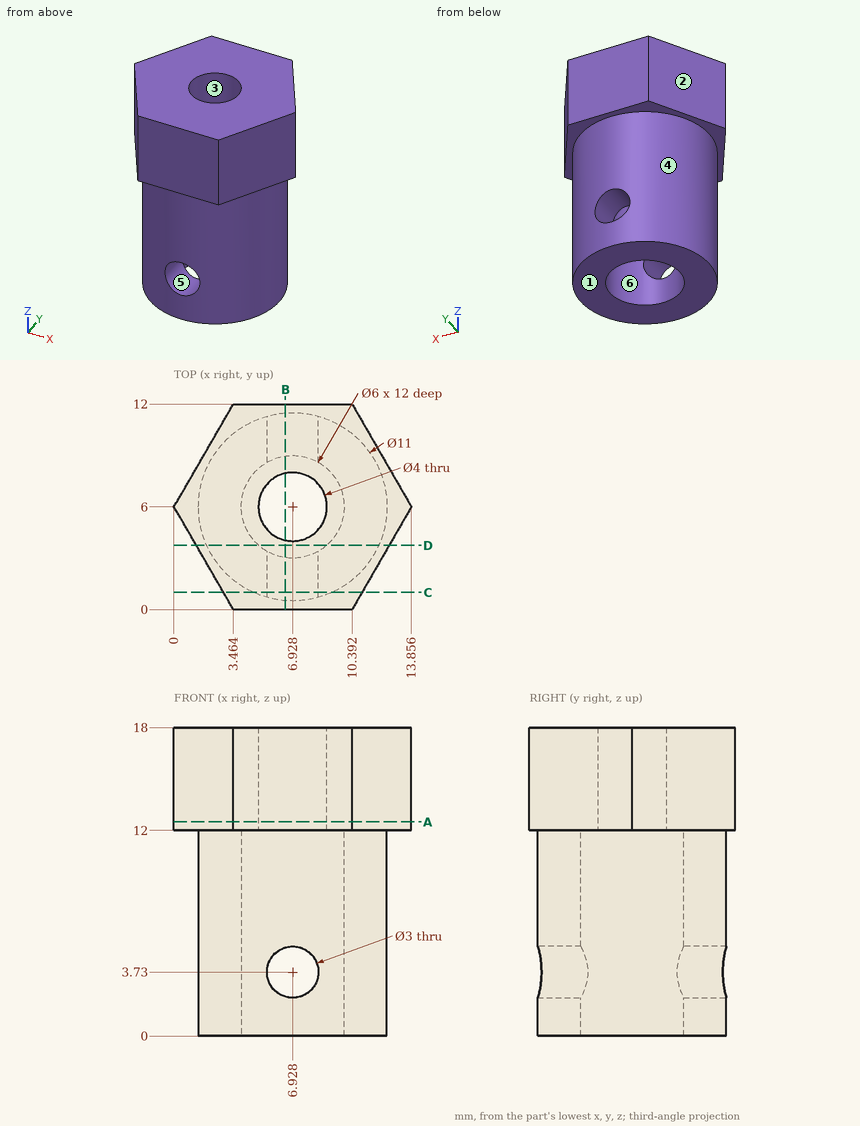
Check sheet for the drawn part. Datum: minimum x, y, z corner. Units: mm. A direction names the side the tool comes from. Give positions to 0.01 mm unless a question says otherwise; leave off trailing zeros. Write each loop counter-clockwise with the first axis right and the second up, starting at its lowest first coordinate (ties: lowest second). Pieces come first, ordered by that corner, then holes.
(1) Material ranges on line 1 (X direction, y = 5, z = 1); line 2 (Z direction, x = 8.25, y = 11); line 3 (Z direction, x = 5.75, y = 11), recorded low to high.
(2) Cross-section at D-D (y = 3.75). Enter the section's corners in (x, z).
(3) Gauge pin test, flat ends, axial feed: pin 1 (5 mm diameter, centred on x = 6.93, y = 6, fed in from -Z); pin 2 (5 mm diameter, centred on x = 6.93, z = 3.73, fed in from -Y); pin 3 (3 mm diameter, centred on y = 7, z = 16, fed in from -X); pin 4 (3.5 mm diameter, centred on x = 6.93, y = 6, fed in from +Z). Record the tip position at first contact, or that the pin passes through.
(4) Mould release check, pull along X, two halves, no side actions. Record for the marked faces 1, 2, 3 and 4: +X half, -X half, draft (parallel to the pull), parting line (faces both ways), or undercut.
(5) Cross-section at C-C (y = 1). Enter the section's corners in (x, z).
(6) Cross-section at A-A (z = 12.5). Enter the section's corners in (x, y), plus the area to 3 significant figures.
(7) Cross-section at B-B (x = 6.5). Enter the section's corners in (y, z).
(8) Access from +Z, -Z, +X, -X, +Y, -Y to the whole of each face (thin tool, end or side, straight path). Record for the marked faces 5 and 6.
Worked out:
1. line 1: x = 1.52 to 4.1, 9.76 to 12.34
1. line 2: z = 0 to 3.02, 4.44 to 18
1. line 3: z = 0 to 2.8, 4.66 to 18
2. outline: (1.3, 12) - (1.91, 12) - (1.91, 0) - (4.94, 0) - (4.94, 12) - (8.91, 12) - (8.91, 0) - (11.95, 0) - (11.95, 12) - (12.56, 12) - (12.56, 18) - (1.3, 18) - close
3. pin 1: stops at z = 12
3. pin 2: stops at y = 0.5
3. pin 3: stops at x = 0
3. pin 4: passes through
4. face 1: draft
4. face 2: -X half
4. face 3: undercut
4. face 4: parting line
5. outline: (2.89, 12) - (4.64, 12) - (4.64, 0) - (9.22, 0) - (9.22, 12) - (10.97, 12) - (10.97, 18) - (2.89, 18) - close; hole circle Ø3 at (6.93, 3.73)
6. outline: (0, 6) - (3.46, 0) - (10.39, 0) - (13.86, 6) - (10.39, 12) - (3.46, 12) - close; hole circle Ø4 at (6.93, 6)
6. area: 112 mm2
7. outline: (0, 12) - (0.52, 12) - (0.52, 5.17) - (3.03, 5.17) - (3.03, 12) - (4.05, 12) - (4.05, 18) - (0, 18) - close; (0.52, 0) - (3.03, 0) - (3.03, 2.29) - (0.52, 2.29) - close; (7.95, 12) - (8.97, 12) - (8.97, 5.17) - (11.48, 5.17) - (11.48, 12) - (12, 12) - (12, 18) - (7.95, 18) - close; (8.97, 0) - (11.48, 0) - (11.48, 2.29) - (8.97, 2.29) - close
8. face 5: +Y, -Y
8. face 6: -Z
